```python
from build123d import *

# Parameters (mm, degrees)
F0_R     = 4.1
F1_DEPTH = 1.9


with BuildPart() as f1:
    # F0 (on Top) → F1 (new body)
    with BuildSketch(Plane.XY):
        with BuildLine():
            Line((3.55, -90), (40.611275, -90))
            Line((40.611275, -90), (44.5, -85.863031))
            Line((44.5, -85.863031), (44.5, -66))
            Line((44.5, -66), (59.422746, -66))
            Line((59.422746, -66), (62.5, -62.361009))
            Line((62.5, -62.361009), (62.5, 62.361009))
            Line((62.5, 62.361009), (59.422746, 66))
            Line((59.422746, 66), (44.5, 66))
            Line((44.5, 66), (44.5, 85.863031))
            Line((44.5, 85.863031), (40.611275, 90))
            Line((40.611275, 90), (3.55, 90))
            Line((3.55, 90), (3.55, 75.3))
            ThreePointArc((3.55, 75.3), (0, 71.75), (-3.55, 75.3))
            Line((-3.55, 75.3), (-3.55, 90))
            Line((-3.55, 90), (-40.611275, 90))
            Line((-40.611275, 90), (-44.5, 85.863031))
            Line((-44.5, 85.863031), (-44.5, 66))
            Line((-44.5, 66), (-59.422746, 66))
            Line((-59.422746, 66), (-62.5, 62.361009))
            Line((-62.5, 62.361009), (-62.5, -62.361009))
            Line((-62.5, -62.361009), (-59.422746, -66))
            Line((-59.422746, -66), (-44.5, -66))
            Line((-44.5, -66), (-44.5, -85.863031))
            Line((-44.5, -85.863031), (-40.611275, -90))
            Line((-40.611275, -90), (-3.55, -90))
            Line((-3.55, -90), (-3.55, -75.3))
            ThreePointArc((-3.55, -75.3), (0, -71.75), (3.55, -75.3))
            Line((3.55, -75.3), (3.55, -90))
        make_face()
        with Locations((-52, -48)):
            Circle(F0_R, mode=Mode.SUBTRACT)
        with Locations((52, -48)):
            Circle(F0_R, mode=Mode.SUBTRACT)
        with Locations((-52, 48)):
            Circle(F0_R, mode=Mode.SUBTRACT)
        with Locations((52, 48)):
            Circle(F0_R, mode=Mode.SUBTRACT)
    extrude(amount=F1_DEPTH)


solid = f1.part
```
CAD build for the part. Positions are in the model's coordinates, mm. Round coordinates to 2 decimals unless told otherwise and drop trailing zeros. Loops run counter-clockwise (first coordinate to the right, second up) from the corner with the lowest first, then second, coordinate; pieces in that order, holes last. Notation, with made-up numbers: M 55.25,84.5 L 99.25,84.5 A19 cw 99.25,113.5 Z; hole C 25.25,34.5 d7. An arc over 180 degrees is marked long. Use a Markdown table: item, result. Add a question column.
(1) Cut at C-C (x = 52). Give the cut face in (y, z), and give its area (3 significant figures).
(2) Drill centre lines: line 1 (Y direction, x = 52, z = 0.45); line 2 (X direction, y = -77, z = 1); line 3 (Y direction, x = 55.5, z = 0.75). Where is each one in solid material? Low to high.
(3) Cut at B-B (y = -48). Give the cut face in (x, z).
(4) Cut at A-A (z = 1.6). State how many separate pieces and enclosed holes the cut face has, and give its area (3 significant figures).
(5) Pull direction Y, two halves, no side cores. Call faces 1 (the face through (-1, 1, 1.9)), 2 (the face through (-0.08, -71.75, 0.94)), 3 (the face through (48.978, 50.771, 0.937)): +Y half, -Y half, draft (parallel to the pull), parting line (faces both ways), or undercut.
(6) Flat gauge pins, fed straight in: pin 1 (13 mm diameter, centred on x = -52, y = 48, fed in from +Z); pin 2 (0.6 mm diameter, centred on y = 86, z = 0.5, fed in from -X); pin 3 (1 mm diameter, centred on x = 53.5, z = 1.5, fed in from -Y); pin 4 (0.6 mm diameter, centred on x = 53, z = 1.5, fed in from +Y). Where does each tip first touch, or does it go through?
Geometry says:
| question | item | result |
|---|---|---|
| 1 | outline | M -66,0 L -52.1,0 L -52.1,1.9 L -66,1.9 Z; M -43.9,0 L 43.9,0 L 43.9,1.9 L -43.9,1.9 Z; M 52.1,0 L 66,0 L 66,1.9 L 52.1,1.9 Z |
| 1 | area | 220 mm² |
| 2 | line 1 | y = -66 to -52.1, -43.9 to 43.9, 52.1 to 66 |
| 2 | line 2 | x = -44.5 to -3.55, 3.55 to 44.5 |
| 2 | line 3 | y = -66 to -50.14, -45.86 to 45.86, 50.14 to 66 |
| 3 | outline | M -62.5,0 L -56.1,0 L -56.1,1.9 L -62.5,1.9 Z; M -47.9,0 L 47.9,0 L 47.9,1.9 L -47.9,1.9 Z; M 56.1,0 L 62.5,0 L 62.5,1.9 L 56.1,1.9 Z |
| 4 | separate pieces | 1 |
| 4 | enclosed holes | 4 |
| 4 | area | 20,300 mm² |
| 5 | face 1 | draft |
| 5 | face 2 | -Y half |
| 5 | face 3 | undercut |
| 6 | pin 1 | stops at z = 1.9 |
| 6 | pin 2 | stops at x = -44.5 |
| 6 | pin 3 | stops at y = -66 |
| 6 | pin 4 | stops at y = 66 |
